Could you check a few things on this model? Use its own coordinates, in mm. Face numbers are marked on the shaded views. A direction names the side the tool comes from. Round coordinates to 2 decimals unless told otherwise and drop trailing zeros. Write each loop counter-clockwise with the first axis right and the second up, starting at its lowest first coordinate (ties: lowest second). Pieces come first, ordered by that corner, then holes. Notation, with made-up numbers: (47, 24) -> (69, 24) arc R21 cw to (69, 42) -> close; hole circle Ø3 at (64, 37.5). An arc over 180 degrees is marked (long way). Answer as CSV lines item,"result". Start each with the question number.
Q1. Imagine slicing it at A-A on z = 12.7. Please give me the cut outline in (x, y), and give its area (3 significant figures).
Q2. Imagine slicing it at D-D on x = -10.5. Please give me the cut outline in (y, z), and give its area (3 significant figures).
Q3. If I drill on line 1 (X direction, y = -16.5, z = 12.7); line 2 (X direction, y = 10.5, z = 19); line 3 (Y direction, x = 1, z = 9.5), over which ranges is the centre line in solid material (lowest first)? Write a range as [from, to].
Q4. Imagine slicing it at C-C on z = 19.5. Please give me the cut outline in (x, y), and give its area (3 significant figures).
Q5. Imagine slicing it at B-B on y = 6. Please give me the cut outline in (x, z), and give its area (3 significant figures).
Q6. Will these pins go through, and if not, where does the flat tip stop? pin 1 Ø12 at (x, y) = (-2, -3) entering from +Z; pin 2 Ø1.5 at (x, z) = (-13, 18) entering from +Y; pin 3 Ø7.5 at (y, z) = (1, 7) entering from +X; pin 4 Ø5 at (y, z) = (-4.5, 13.5) entering from -X.
Q7. If we mould it in two halves opening along Z, with no side actions, what happens to the marked faces 1, 2 and 3? For each: pulls with the +Z half, pulls with the -Z half, needs draft (parallel to the pull), parting line crosses it, or undercut.
Q8. For the marked faces 4 and 5, which set-ups out of +Z, -Z, +X, -X, +Y, -Y let a thin tool reach every point of the face, with its end or its side?
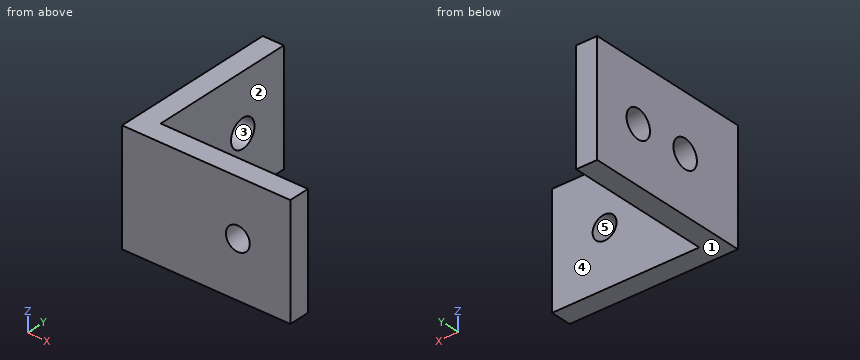
from build123d import *

# Parameters (mm, degrees)
BOSS_EXTRUDE1_DEPTH     = 25.4
CUT_EXTRUDE1_REACH      = 51.636
SKETCH2_R               = 3.175
F_1_4_28_TAPPED_HOLE1_D = 5.4102


with BuildPart() as part:
    # Sketch1 → Boss-Extrude1 (new body)
    with BuildSketch(Plane.XY):
        Polygon((-23.771121012, 18.943273067), (-23.771121012, -19.156726933), (14.328878988, -19.156726933), (14.328878988, -14.394226933), (-19.008621012, -14.394226933), (-19.008621012, 18.943273067), align=None)
    extrude(amount=BOSS_EXTRUDE1_DEPTH)

    # Sketch2 → Cut-Extrude1 (cut, up to next)
    with BuildSketch(Plane.ZY.offset(23.771121012), mode=Mode.PRIVATE) as cut_extrude1_sk1:
        with Locations(Location((12.7, 7.830773067, 0), (0, 0, 270))):
            Circle(SKETCH2_R)
    cut_extrude1_tool1 = extrude(cut_extrude1_sk1.sketch, amount=-CUT_EXTRUDE1_REACH, mode=Mode.PRIVATE) & part.part
    # Sketch2 → Cut-Extrude1 (cut, up to next)
    with BuildSketch(Plane.ZY.offset(23.771121012), mode=Mode.PRIVATE) as cut_extrude1_sk2:
        with Locations(Location((12.7, -4.869226933, 0), (0, 0, 270))):
            Circle(SKETCH2_R)
    cut_extrude1_tool2 = extrude(cut_extrude1_sk2.sketch, amount=-CUT_EXTRUDE1_REACH, mode=Mode.PRIVATE) & part.part
    add(cut_extrude1_tool1.solids().sort_by_distance((-23.771121, 7.830773, 12.7))[0], mode=Mode.SUBTRACT)
    add(cut_extrude1_tool2.solids().sort_by_distance((-23.771121, -4.869227, 12.7))[0], mode=Mode.SUBTRACT)

    # 1/4-28 Tapped Hole1 (through all)
    with Locations(Plane(origin=(0, -19.156726933, 0), x_dir=(-1, 0, 0), z_dir=(0, -1, 0))):
        with Locations((-2.441678988, -12.7)):
            Hole(F_1_4_28_TAPPED_HOLE1_D / 2)


solid = part.part
Checks:
1,outline,"(-23.77, -19.16) -> (-0.26, -19.16) -> (-0.26, -14.39) -> (-19.01, -14.39) -> (-19.01, -8.04) -> (-23.77, -8.04) -> close; (-23.77, -1.69) -> (-19.01, -1.69) -> (-19.01, 4.66) -> (-23.77, 4.66) -> close; (-23.77, 11.01) -> (-19.01, 11.01) -> (-19.01, 18.94) -> (-23.77, 18.94) -> close; (5.15, -19.16) -> (14.33, -19.16) -> (14.33, -14.39) -> (5.15, -14.39) -> close"
1,area,"254 mm^2"
2,outline,"(-19.16, 0) -> (-14.39, 0) -> (-14.39, 25.4) -> (-19.16, 25.4) -> close"
2,area,"121 mm^2"
3,line 1,"[-23.77, -0.26], [5.15, 14.33]"
3,line 2,"[-23.77, -19.01]"
3,line 3,"[-19.16, -14.39]"
4,outline,"(-23.77, -19.16) -> (14.33, -19.16) -> (14.33, -14.39) -> (-19.01, -14.39) -> (-19.01, 18.94) -> (-23.77, 18.94) -> close"
4,area,"340 mm^2"
5,outline,"(-23.77, 0) -> (-19.01, 0) -> (-19.01, 10.11) -> (-23.77, 10.11) -> close; (-23.77, 15.29) -> (-19.01, 15.29) -> (-19.01, 25.4) -> (-23.77, 25.4) -> close"
5,area,"96.3 mm^2"
6,pin 1,"through"
6,pin 2,"y = -14.39"
6,pin 3,"x = -19.01"
6,pin 4,"x = -23.77"
7,face 1,"pulls with the -Z half"
7,face 2,"needs draft"
7,face 3,"undercut"
8,face 4,"+Z, -Z, +X, +Y"
8,face 5,"+Y, -Y"
